The listing builds one solid part. Answer for the finished solid, in the listing's coordinates (mm). A direction names the side the tool comes from. Round coordinates to 2 decimals unless told otherwise and drop trailing zeros. Order: outer loops, then holes, each group sorted by start corner. A loop starts at its lowest first (then second) coordinate and runs counter-clockwise, first axis right, second up. Notation, with made-up numbers: (2.25, 1) -> (16.25, 1) arc R27 ccw to (16.25, 29) -> close; hole circle Ø1 at (14, 65.25). An arc over 180 degrees is marked (long way). Return JSON: item names as keys, results as strings. Group by question number.
(1) Consider line 1 (Y direction, x = 0, z = 1.15); line 2 (X direction, y = 0, z = 0.55) (3 decimals); line 3 (Z direction, x = -2, y = 6). Determine where each line is inside the solid, lowest interval first. Write a range as [from, to].
(2) Each of these flat-tipped pins is pushed along its axis until it touches: pin 1 (2 mm diameter, centred on x = -2.5, z = 0, fed in from +Y); pin 2 (1 mm diameter, centred on y = 9, z = 12.5, fed in from -X); pin 3 (2 mm diameter, centred on x = 0, z = 5, fed in from -Y); pin 4 (4 mm diameter, centred on x = 3.5, z = 11, fed in from +Y). Where does it stop, or does it pass through?
(3) Which of the six approach directions +Z, -Z, +X, -X, +Y, -Y give full straight-line access (tool end or side, diameter ignored) to faces 1 (the face through (6.691, 12.864, 0.986)), 2 (the face through (0, -14, 4.7)), 3 (the face through (1.91, 3.37, 0.52)), 4 (the face through (-14.985, 0.66, 10.359))?
(4) Determine the mould class of faces 5 (the face through (12.932, 5.362, -4.311)), 6 (the face through (-0.6, -20.35, 5)), 7 (the face through (1.965, -3.34, 0.521)) for opening direction X: +X half, -X half, draft (parallel to the pull), parting line (faces both ways), or undercut.
(5) The part is cut by section C-C (z = 11). Determine the outline of the cut face in (x, y), plus the area to 3 significant figures.
(6) The part is cut by section B-B (z = 5). Determine the outline of the cut face in (x, y) (3 decimals).
from build123d import *

# Parameters (mm, degrees)
F0_R      = 15
F1_DEPTH  = 19
F2_R      = 1.5875
F3_R      = 15.5
F3_R_2    = 15
F4_DEPTH  = 3.5
F5_R      = 14.5
F6_DEPTH  = 2
F8_DEPTH  = 3
F9_R      = 5.75
F10_DEPTH = 2
F11_R     = 14
F11_R_2   = 5.75
F12_DEPTH = 2.66
F14_START = 14
F13_R     = 1.375
F14_DEPTH = 11.4
F15_R     = 0.5
F16_DEPTH = 6.35


with BuildPart() as f1:
    # F0 (on Top) → F1 (new body)
    with BuildSketch(Plane.XY):
        Circle(F0_R)
    extrude(amount=F1_DEPTH)

    # F2
    f2_edges = [f1.edges().sort_by_distance(p)[0] for p in [
        (-15, 0, 19),
    ]]
    fillet(f2_edges, radius=F2_R)

    # F3 (on face) → F4 (join)
    with BuildSketch(Plane(origin=(0, 0, 0), x_dir=(1, 0, 0), z_dir=(0, 0, -1))):
        Circle(F3_R)
        Circle(F3_R_2, mode=Mode.SUBTRACT)
    extrude(amount=-F4_DEPTH)

    # F5 (on face) → F6 (cut)
    with BuildSketch(Plane(origin=(0, 0, 0), x_dir=(1, 0, 0), z_dir=(0, 0, -1))):
        Circle(F5_R)
    extrude(amount=-F6_DEPTH, mode=Mode.SUBTRACT)

    # F7 (on face) → F8 (join)
    with BuildSketch(Plane(origin=(0, 0, 2), x_dir=(1, 0, 0), z_dir=(0, 0, -1))):
        Polygon((0, 4.4744645862), (-3.875, 2.2372322931), (-3.875, -2.2372322931), (0, -4.4744645862), (3.875, -2.2372322931), (3.875, 2.2372322931), align=None)
    extrude(amount=F8_DEPTH)

    # F9 (on face) → F10 (join)
    with BuildSketch(Plane(origin=(0, 0, -1), x_dir=(1, 0, 0), z_dir=(0, 0, -1))):
        Circle(F9_R)
        Polygon((-3.875, 2.2372322931), (0, 4.4744645862), (3.875, 2.2372322931), (3.875, -2.2372322931), (0, -4.4744645862), (-3.875, -2.2372322931), align=None, mode=Mode.SUBTRACT)
        Polygon((3.875, 2.2372322931), (0, 4.4744645862), (-3.875, 2.2372322931), (-3.875, -2.2372322931), (0, -4.4744645862), (3.875, -2.2372322931), align=None)
    extrude(amount=F10_DEPTH)

    # F11 (on face) → F12 (join)
    with BuildSketch(Plane(origin=(0, 0, -3), x_dir=(1, 0, 0), z_dir=(0, 0, -1))):
        Circle(F11_R)
        Circle(F11_R_2, mode=Mode.SUBTRACT)
        Circle(F11_R_2)
    extrude(amount=F12_DEPTH)

    # F13 (on Front) → F14 (cut)
    with BuildSketch(Plane.XZ.offset(F14_START)):
        with Locations((0, 5)):
            Circle(F13_R)
    extrude(amount=F14_DEPTH, mode=Mode.SUBTRACT)

    # F15 (on face) → F16 (join)
    with BuildSketch(Plane.XZ.offset(14)):
        with Locations((-0.635, 5)):
            Circle(F15_R)
        with Locations((0.635, 5)):
            Circle(F15_R)
    extrude(amount=F16_DEPTH)


solid = f1.part
Answer below:
{
 "1": {"line 1": "y = [-15.5, -14.5], [-4.47, 4.47], [14.5, 15.5]", "line 2": "x = [-15.5, -14.5], [-3.875, 3.875], [14.5, 15.5]", "line 3": "z = [-5.66, -3], [2, 19]"},
 "2": {"pin 1": "stops at y = 15.43", "pin 2": "stops at x = -12.36", "pin 3": "stops at y = -20.35", "pin 4": "stops at y = 14.92"},
 "3": {"face 1": "-Z", "face 2": "-Y", "face 3": "none", "face 4": "+Z"},
 "4": {"face 5": "parting line", "face 6": "draft", "face 7": "undercut"},
 "5": {"outline": "circle Ø30 at (0, 0)", "area": "707 mm²"},
 "6": {"outline": "(-1.375, -14.937) -> (-1.375, -14) -> (-1.135, -14) -> (-1.135, -20.35) -> (-0.135, -20.35) -> (-0.135, -14) -> (0.135, -14) -> (0.135, -20.35) -> (1.135, -20.35) -> (1.135, -14) -> (1.375, -14) -> (1.375, -14.937) arc R15 ccw (long way) to start"}
}
